Build history of the part. All positions in model axes, mm. Coordinates: 2 decimals unless noted, no trailing zeros. Loops run counter-clockwise (first coordinate to the right, second up) from the corner with the lowest first, then second, coordinate; pieces in that order, holes last. Notation, with made-up numbers: (4.5, -35) - (44.5, -35) arc R11 ccw to (44.5, -26) - close; hole circle Ø5 at (74.5, -9.5). An arc over 180 degrees is marked (long way). One line per item, written item: value.
```python
from build123d import *

# Parameters (mm, degrees)
F0_R     = 10
F0_R_2   = 1.5
F1_DEPTH = 1


with BuildPart() as f1:
    # F0 (on Front) → F1 (new body, symmetric)
    with BuildSketch(Plane.XZ):
        Circle(F0_R)
        with BuildLine():
            ThreePointArc((-4.548809, -5.320558), (-4.894761, -4.468726), (-4.398979, -3.694453))
            Line((-4.398979, -3.694453), (-2.5, -2.598076))
            ThreePointArc((-2.5, -2.598076), (-2, -2.464102), (-1.5, -2.598076))
            ThreePointArc((-1.5, -2.598076), (0, -3), (1.5, -2.598076))
            ThreePointArc((1.5, -2.598076), (2, -2.464102), (2.5, -2.598076))
            Line((2.5, -2.598076), (4.398979, -3.694453))
            ThreePointArc((4.398979, -3.694453), (4.894761, -4.468726), (4.548809, -5.320558))
            ThreePointArc((4.548809, -5.320558), (0, -7), (-4.548809, -5.320558))
        make_face(mode=Mode.SUBTRACT)
        with BuildLine():
            ThreePointArc((-6.882143, -1.279106), (-6.062178, 3.5), (-2.333333, 6.599663))
            ThreePointArc((-2.333333, 6.599663), (-1.42265, 6.473351), (-1, 5.656854))
            Line((-1, 5.656854), (-1, 3.464102))
            ThreePointArc((-1, 3.464102), (-1.133975, 2.964102), (-1.5, 2.598076))
            ThreePointArc((-1.5, 2.598076), (-2.598076, 1.5), (-3, 0))
            ThreePointArc((-3, 0), (-3.133975, -0.5), (-3.5, -0.866025))
            Line((-3.5, -0.866025), (-5.398979, -1.962402))
            ThreePointArc((-5.398979, -1.962402), (-6.317411, -2.004625), (-6.882143, -1.279106))
        make_face(mode=Mode.SUBTRACT)
        Circle(F0_R_2, mode=Mode.SUBTRACT)
        with BuildLine():
            Line((1, 3.464102), (1, 5.656854))
            ThreePointArc((1, 5.656854), (1.42265, 6.473351), (2.333333, 6.599663))
            ThreePointArc((2.333333, 6.599663), (6.062178, 3.5), (6.882143, -1.279106))
            ThreePointArc((6.882143, -1.279106), (6.317411, -2.004625), (5.398979, -1.962402))
            Line((5.398979, -1.962402), (3.5, -0.866025))
            ThreePointArc((3.5, -0.866025), (3.133975, -0.5), (3, 0))
            ThreePointArc((3, 0), (2.598076, 1.5), (1.5, 2.598076))
            ThreePointArc((1.5, 2.598076), (1.133975, 2.964102), (1, 3.464102))
        make_face(mode=Mode.SUBTRACT)
    extrude(amount=F1_DEPTH, both=True)

    # F2 (on Right) → F3 (revolve, cut)
    with BuildSketch(Plane.YZ):
        Polygon((-0.75, 10), (0, 8.5), (0, 10), align=None)
        Polygon((0, 10), (0, 8.5), (0.75, 10), align=None)
    revolve(axis=Axis((0, -0.781199, 0), (0, -1, 0)), mode=Mode.SUBTRACT)


solid = f1.part
```
Item 1: Cut at A-A, the plane x = 0. Write the cut outline in (y, z), then the cut area to 4 significant figures.
Check result:
outline: (-1, -10) - (-0.75, -10) - (0, -8.5) - (0.75, -10) - (1, -10) - (1, -7) - (-1, -7) - close; (-1, -3) - (1, -3) - (1, -1.5) - (-1, -1.5) - close; (-1, 1.5) - (1, 1.5) - (1, 10) - (0.75, 10) - (0, 8.5) - (-0.75, 10) - (-1, 10) - close
area: 23.75 mm^2
Item 2: Probe probe 1 along X at (y, z) = (0.45, 4.5); probe 2 along X at (y, z) = (-0.3, -2); probe 3 along Z at (x, y) = (2.25, 0.4). List the from-to ranges inside material, lowest first. Write a range as from..to.
Check result:
probe 1: x = -8.25..-5.36, -1..1, 5.36..8.25
probe 2: x = -8.88..-6.33, -5.47..5.47, 6.33..8.88
probe 3: z = -9.02..-6.63, -2.5..1.98, 6.63..9.02
Item 3: Cut at B-B, the plane y = 0.4. Write the cut outline in (x, z).
Check result:
outline: circle Ø18.6 at (0, 0); hole (-6.88, -1.28) arc R1 ccw to (-5.4, -1.96) - (-3.5, -0.87) arc R1 ccw to (-3, 0) arc R3 cw to (-1.5, 2.6) arc R1 ccw to (-1, 3.46) - (-1, 5.66) arc R1 ccw to (-2.33, 6.6) arc R7 ccw to start; hole (-4.55, -5.32) arc R7 ccw to (4.55, -5.32) arc R1 ccw to (4.4, -3.69) - (2.5, -2.6) arc R1 ccw to (1.5, -2.6) arc R3 cw to (-1.5, -2.6) arc R1 ccw to (-2.5, -2.6) - (-4.4, -3.69) arc R1 ccw to start; hole circle Ø3 at (0, 0); hole (1, 3.46) arc R1 ccw to (1.5, 2.6) arc R3 cw to (3, 0) arc R1 ccw to (3.5, -0.87) - (5.4, -1.96) arc R1 ccw to (6.88, -1.28) arc R7 ccw to (2.33, 6.6) arc R1 ccw to (1, 5.66) - close
Item 4: Drop a flat-ended pin along its axis: P1, Ø1, axis at y = 0.5, z = -7, coming from the -X side. Give the stop position or say it passes through.
Check result:
P1: stops at x = -7.54
Item 5: Cut at C-C, the plane z = 3. Give the number of separate pieces and of enclosed holes in the cut face, then the cut area to 3 significant figures.
Check result:
separate pieces: 3
enclosed holes: 0
area: 14.9 mm^2
Item 6: Pull direction X, two halves, no side cores. Call faces 1 (the face through (1, 0, 5)), 2 (the face through (2, -1, 0)): released by +X, released by -X, zero draft, split by the parting line, or undercut.
Check result:
face 1: undercut
face 2: zero draft
